Could you check a few things on this model? Use its own coordinates, in mm. A direction names the side the tool comes from. Coordinates: 2 decimals unless noted, no trailing zeros. Write each loop counter-clockwise with the first axis right and the second up, starting at its lowest first coordinate (ties: lowest second). Pieces come first, ordered by that corner, then holes. Notation, with made-up numbers: (33, -27.75) - (68, -27.75) arc R24 ccw to (68, 4.25) - close; hole circle Ø2 at (30.5, 6.25). An arc over 180 degrees is marked (long way). Write item = value, one per line. Start each with the question number.
```python
from build123d import *

# Parameters (mm, degrees)
F0_W      = 69.85
F0_H      = 38.1
F1_DEPTH  = 25.4
F2_W      = 44.45
F2_H      = 25.4
F3_DEPTH  = 25.4
F5_DEPTH  = 25.4
F7_DEPTH  = 25.4
F8_R      = 6.7378707766
F9_DEPTH  = 25.4
F11_DEPTH = 25.4


with BuildPart() as f1:
    # F0 (on Front) → F1 (new body)
    with BuildSketch(Plane.XZ):
        with Locations((34.925, 19.05)):
            Rectangle(F0_W, F0_H)
    extrude(amount=-F1_DEPTH)

    # F2 (on face) → F3 (cut)
    with BuildSketch(Plane.XZ):
        with Locations((47.625, 25.4)):
            Rectangle(F2_W, F2_H)
    extrude(amount=-F3_DEPTH, mode=Mode.SUBTRACT)

    # F4 (on face) → F5 (cut)
    with BuildSketch(Plane.XY.offset(12.7)):
        with BuildLine():
            ThreePointArc((38.1, 6.35), (42.5901280605, 8.2098719395), (44.45, 12.7))
            ThreePointArc((44.45, 12.7), (42.5901280605, 17.1901280605), (38.1, 19.05))
            ThreePointArc((38.1, 19.05), (31.75, 12.7), (38.1, 6.35))
        make_face()
        with BuildLine():
            ThreePointArc((38.1, 19.05), (42.5901280605, 17.1901280605), (44.45, 12.7))
            ThreePointArc((44.45, 12.7), (42.5901280605, 8.2098719395), (38.1, 6.35))
            Line((38.1, 6.35), (57.15, 6.35))
            ThreePointArc((57.15, 6.35), (50.8, 12.7), (57.15, 19.05))
            Line((57.15, 19.05), (38.1, 19.05))
        make_face()
        with BuildLine():
            ThreePointArc((63.5, 12.7), (61.6401280605, 17.1901280605), (57.15, 19.05))
            ThreePointArc((57.15, 19.05), (50.8, 12.7), (57.15, 6.35))
            ThreePointArc((57.15, 6.35), (61.6401280605, 8.2098719395), (63.5, 12.7))
        make_face()
    extrude(amount=-F5_DEPTH, mode=Mode.SUBTRACT)

    # F6 (on face) → F7 (cut)
    with BuildSketch(Plane.XY.offset(12.7)):
        with BuildLine():
            ThreePointArc((57.15, 25.4), (66.1302561211, 21.6802561211), (69.85, 12.7))
            Line((69.85, 12.7), (69.85, 25.4))
            Line((69.85, 25.4), (57.15, 25.4))
        make_face()
        with BuildLine():
            ThreePointArc((69.85, 12.7), (66.1302561211, 3.7197438789), (57.15, 0))
            Line((57.15, 0), (69.85, 0))
            Line((69.85, 0), (69.85, 12.7))
        make_face()
    extrude(amount=-F7_DEPTH, mode=Mode.SUBTRACT)

    # F8 (on face) → F9 (cut)
    with BuildSketch(Plane.XZ):
        with Locations((12.7, 25.4)):
            Circle(F8_R)
    extrude(amount=-F9_DEPTH, mode=Mode.SUBTRACT)

    # F10 (on face) → F11 (cut)
    with BuildSketch(Plane.XZ):
        with BuildLine():
            ThreePointArc((0, 25.4), (3.7197438789, 34.3802561211), (12.7, 38.1))
            Line((12.7, 38.1), (0, 38.1))
            Line((0, 38.1), (0, 25.4))
        make_face()
        with BuildLine():
            ThreePointArc((12.7, 38.1), (21.6802561211, 34.3802561211), (25.4, 25.4))
            Line((25.4, 25.4), (25.4, 38.1))
            Line((25.4, 38.1), (12.7, 38.1))
        make_face()
    extrude(amount=-F11_DEPTH, mode=Mode.SUBTRACT)


solid = f1.part
```
1) For P1, Ø3, axis at x = 36, y = 22, coming from the +Z side; P2, Ø5, axis at x = 48, y = 11, coming from the +Z side; P3, Ø3, axis at x = 32, y = 12.5, coming from the -Z side; P4, Ø8, axis at y = 19.5, z = 30.5, coming from the +X side, each with a flat end and sliding along its axis, tell me the tip position at first contact or that it passes through.
2) Suppose I cut it at D-D on y = 2.5. Please give me the cut outline in (x, z), plus the area to 3 significant figures.
3) Thinking about a two-plate mould opening in Z: for faces 4 (the flat face through (27, 13, 0)), 5 (the flat face through (47, 4, 12.7)), 6 (the cylindrical face through (11.82, 12.52, 32.08)), 7 (the cylindrical face through (31.75, 12.84, 6.44)), which applies, +Z half, -Z half, draft (parallel to the pull), parting line (faces both ways), or undercut?
4) Suppose I cut it at B-B on z = 9. Please give me the cut outline in (x, y).
5) If I drill on probe 1 along Z at (x, y) = (12.7, 10); probe 2 along Z at (x, y) = (27, 10); probe 3 along X at (y, z) = (14, 23), over which ranges is the centre line in solid material (lowest first)? Write a range as [from, to].
6) Suppose I cut it at C-C on x = 8. Please give me the cut outline in (y, z), plus the area to 3 significant figures.
7) Suppose I cut it at A-A on y = 16.75. Please give me the cut outline in (x, z).
8) Which directions (+Z, -Z, +X, -X, +Y, -Y) give clear straight access to the entire face, cutting with the end or side of a thin tool? Please do faces 1 (the flat face through (47, 6.35, 6)), 2 (the flat face through (25.4, 13, 19)), 3 (the flat face through (22, 0, 15)).
Reply:
q1.P1 = 12.7
q1.P2 = through
q1.P3 = 0
q1.P4 = 25.35
q2.outline = (0, 0) - (64.72, 0) - (64.72, 12.7) - (25.4, 12.7) - (25.4, 25.4) arc R12.7 ccw to (0, 25.4) - close; hole circle Ø13.48 at (12.7, 25.4)
q2.area = 1,260 mm^2
q3.face_4 = -Z half
q3.face_5 = +Z half
q3.face_6 = undercut
q3.face_7 = draft
q4.outline = (0, 0) - (57.15, 0) arc R12.7 ccw to (57.15, 25.4) - (0, 25.4) - close; hole (38.1, 6.35) - (57.15, 6.35) arc R6.35 ccw to (57.15, 19.05) - (38.1, 19.05) arc R6.35 ccw to start
q5.probe_1 = [0, 18.66], [32.14, 38.1]
q5.probe_2 = [0, 12.7]
q5.probe_3 = [0, 6.4], [19, 25.4]
q6.outline = (0, 0) - (25.4, 0) - (25.4, 20.57) - (0, 20.57) - close; (0, 30.23) - (25.4, 30.23) - (25.4, 37.2) - (0, 37.2) - close
q6.area = 700 mm^2
q7.outline = (0, 0) - (33.21, 0) - (33.21, 12.7) - (25.4, 12.7) - (25.4, 25.4) arc R12.7 ccw to (0, 25.4) - close; (62.04, 0) - (69.19, 0) - (69.19, 12.7) - (62.04, 12.7) - close; hole circle Ø13.48 at (12.7, 25.4)
q8.face_1 = +Z, -Z
q8.face_2 = +Z, +X, +Y, -Y
q8.face_3 = +Z, -Z, +X, -X, -Y
